Autodesk Inventor part; units mm, degrees
ref_plane "YZ Plane" through (0, 0, 0) normal (1, 0, 0) x (0, 1, 0)
ref_plane "XZ Plane" through (0, 0, 0) normal (0, 1, 0) x (-1, 0, 0)
ref_plane "XY Plane" through (0, 0, 0) normal (0, 0, 1) x (1, 0, 0)
sketch "Náčrt1" plane through (0, 0, 0) normal (0, 1, 0) x (-1, 0, 0)
  line L0 (10, 25) -> (-10, 25)
  line L1 (-10, 25) -> (-10, -25)
  line L2 (-10, -25) -> (10, -25)
  line L3 (10, -25) -> (10, 25)
  line L4 (0, -35) -> (0, 35)
  line L5 (-14, 0) -> (14, 0)
  point P0 (0, 0)
  dimension "d0" = 50
  dimension "d1" = 20
extrude "Vysunutí1" add sketch "Náčrt1" along normal mid plane 1.5
sketch "Náčrt2" plane through (0, 0.75, 0) normal (0, 1, 0) x (1, 0, 0)
  line L0 (-10, -25) -> (10, -25)
  line L1 (10, -25) -> (10, 25)
  line L2 (10, 25) -> (-10, 25)
  point P0 (0, 0)
  point P1 (5, -20)
  point P2 (-5, -20)
  dimension "d4" = 5
  dimension "d5" = 5
  dimension "d6" = 10
  dimension "d7" = 5
hole "Díra1" at (5, 0.75, 20) at (-5, 0.75, 20) direction (0, -1, 0) diameter 3.2 end through all
sketch "Náčrt3" plane through (0, 0.75, 0) normal (0, 1, 0) x (1, 0, 0)
  circle A0 centre (-5, -20) radius 1.6
  circle A1 centre (5, -20) radius 1.6
  line L0 (10, -25) -> (10, 25)
  line L1 (10, 25) -> (-10, 25)
  line L2 (-10, 25) -> (-10, -25)
  line L3 (-10, -25) -> (10, -25)
  point P0 (0, 0)
  point P1 (4, -4)
  point P2 (4, 21)
  dimension "d19" = 4
  dimension "d20" = 6
  dimension "d21" = 6
  dimension "d22" = 25
hole "Díra2" at (4, 0.75, 4) at (4, 0.75, -21) direction (0, -1, 0) diameter 4.5 end through all
properties part number "y_anchor_holder" material "Hliník 6061"
Could you check a few things on this model? Use its own coordinates, in mm. Round coordinates to 2 decimals unless told otherwise and drop trailing zeros. Write each loop counter-clockwise with the first axis right and the second up, starting at its lowest first coordinate (ties: lowest second). Pieces come first, ordered by that corner, then holes. Notation, with made-up numbers: M -10.75,-3.5 L 43.25,-3.5 A28 cw 43.25,14.5 Z; hole C 15,54.5 d3. An arc over 180 degrees is marked long. Answer in a Markdown table with one row per item. Add a question column.
Q1. If I drill on line 1 (X direction, y = -0.4, z = 20); line 2 (Z direction, x = 4.25, y = 0.05); line 3 (Z direction, x = 5.5, y = 0.3), over which ranges is the centre line in solid material (lowest first)? Write a range as from..to.
Q2. Imagine slicing it at B-B (x = -5). Please give me the cut outline in (y, z).
Q3. Imagine slicing it at C-C (z = 4). Please give me the cut outline in (x, y), then the cut area to 4 significant figures.
Q4. Will this pin go through, and if not, where does the flat tip stop? pin 1 Ø4 at (x, z) = (4, 4) entering from +Y.
Q5. Imagine slicing it at D-D (y = -0.05). Please give me the cut outline in (x, z).
Q6. Imagine slicing it at A-A (z = 20). Please give me the cut outline in (x, y).
Values:
| question | item | result |
|---|---|---|
| 1 | line 1 | -10..-6.6, -3.4..3.4, 6.6..10 |
| 1 | line 2 | -25..-23.24, -18.76..1.76, 6.24..18.59, 21.41..25 |
| 1 | line 3 | -25..-22.68, -19.32..2.32, 5.68..18.48, 21.52..25 |
| 2 | outline | M -0.75,-25 L 0.75,-25 L 0.75,18.4 L -0.75,18.4 Z; M -0.75,21.6 L 0.75,21.6 L 0.75,25 L -0.75,25 Z |
| 3 | outline | M -10,-0.75 L 1.75,-0.75 L 1.75,0.75 L -10,0.75 Z; M 6.25,-0.75 L 10,-0.75 L 10,0.75 L 6.25,0.75 Z |
| 3 | area | 23.25 mm^2 |
| 4 | pin 1 | through |
| 5 | outline | M -10,-25 L 10,-25 L 10,25 L -10,25 Z; hole C -5,20 d3.2; hole C 4,-21 d4.5; hole C 4,4 d4.5; hole C 5,20 d3.2 |
| 6 | outline | M -10,-0.75 L -6.6,-0.75 L -6.6,0.75 L -10,0.75 Z; M -3.4,-0.75 L 3.4,-0.75 L 3.4,0.75 L -3.4,0.75 Z; M 6.6,-0.75 L 10,-0.75 L 10,0.75 L 6.6,0.75 Z |
